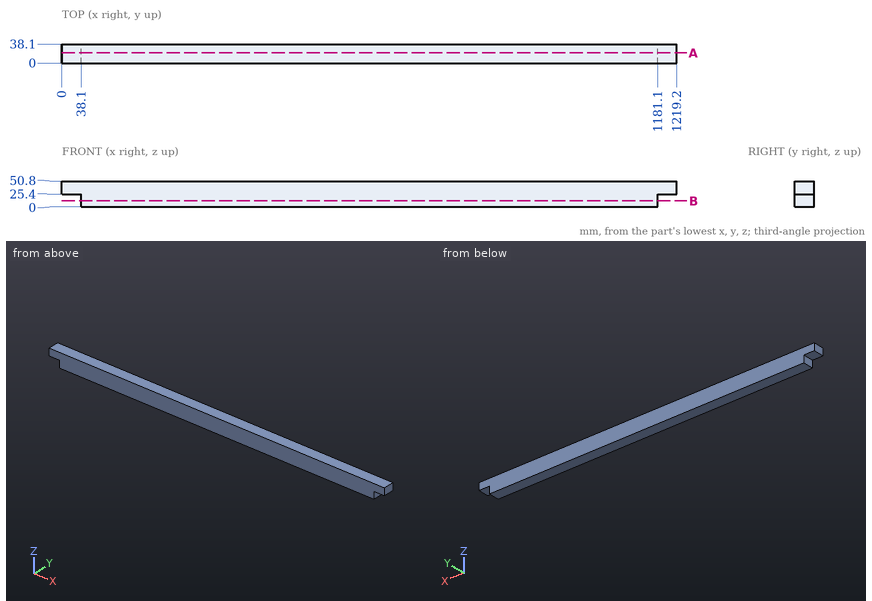
Print and shaded views of the part. All mm, measured from the part's lowest x, y and z. Round coordinates to 2 decimals unless told otherwise and drop trailing zeros. Write each loop counter-clockwise with the first axis right and the second up, starting at its lowest first coordinate (ties: lowest second). Pieces come first, ordered by that corner, then holes. Notation, with made-up numbers: (62.5, 3.5) -> (80.5, 3.5) arc R11 cw to (80.5, 15.5) -> close; hole circle Ø8 at (37.5, 77.5). An arc over 180 degrees is marked (long way). Answer in a Markdown table with one row per item. Add a question column.
Item 1: Saw through at B-B, the plane z = 12. Write the cut outline in (x, y), then the cut area to 3 significant figures.
Item 2: Drop flat-ended pins along their axis: pin 1 Ø11.5 at (x, y) = (9.5, 11) entering from -Z; pin 2 Ø2 at (y, z) = (13.5, 16.5) entering from -X. Give the stop position or say it passes through.
Item 3: Saw through at A-A, the plane y = 20.5. Write the cut outline in (x, z), then the cut area to 3 significant figures.
Item 4: Drill centre line: line 1 (X direction, y = 5.5, z = 7.5). Where is it in solid material? Low to high. Write a range as from..to.
Findings below:
| question | item | result |
|---|---|---|
| 1 | outline | (38.1, 0) -> (1181.1, 0) -> (1181.1, 38.1) -> (38.1, 38.1) -> close |
| 1 | area | 43,500 mm^2 |
| 2 | pin 1 | stops at z = 25.4 |
| 2 | pin 2 | stops at x = 38.1 |
| 3 | outline | (0, 25.4) -> (38.1, 25.4) -> (38.1, 0) -> (1181.1, 0) -> (1181.1, 25.4) -> (1219.2, 25.4) -> (1219.2, 50.8) -> (0, 50.8) -> close |
| 3 | area | 60,000 mm^2 |
| 4 | line 1 | x = 38.1..1181.1 |
